Verification items for this drawing (mm, ordinates from the low corner). A direction names the side the tool comes from. Give positions to 0.01 mm unless a question says otherwise; leave off trailing zeros. Order: outer loops, then holes, each group sorted by start corner. A loop starts at its lowest first (then second) coordinate and runs counter-clockwise, first axis right, second up.
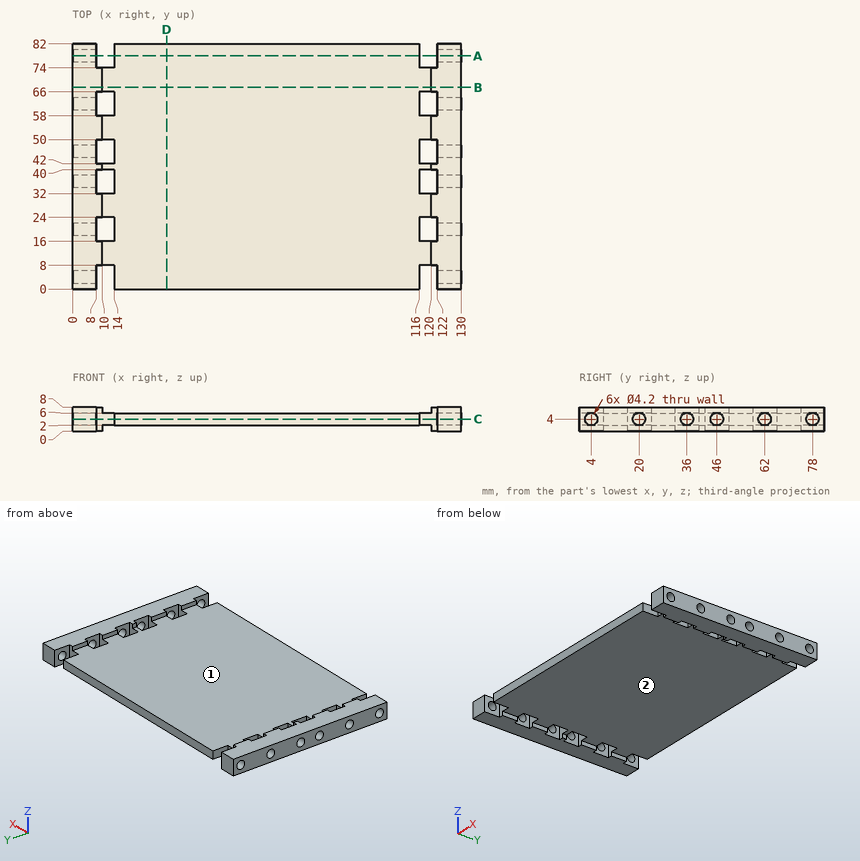
Q1. Cross-section at A-A, the plane y = 78. Record the boundary of the cut face in (x, z), and give its area (3 significant figures).
Q2. Thickness scan on L1, parallel to X at y = 49, z = 2.5; L2, parallel to Y at x = 10.5, z = 4; L3, parallel to X at y = 44, z = 6.5. Record the ranges inside material, lowest first.
Q3. Gauge pin test, flat ends, axial feed: P1, Ø4.5, axis at y = 61, z = 5, coming from the +X side; P2, Ø12, axis at x = 41, y = 22.5, coming from the +Z side; P3, Ø3, axis at y = 20, z = 3.5, coming from the -X side; P4, Ø3, axis at x = 11, z = 2.5, coming from the +Y side. Record the tip position at first contact, or that the pin passes through.
Q4. Cross-section at C-C, the plane z = 4. Give the number of separate pieces and of enclosed holes in the cut face, and give its area (3 significant figures).
Q5. Access from +Z, -Z, +X, -X, +Y, -Y to the whole of each face (thin tool, end or side, straight path). Record for the marked faces 1 and 2.
Q6. Cross-section at B-B, the plane y = 67.5. Record the boundary of the cut face in (x, z).
Q7. Cross-section at D-D, the plane x = 31.5. Record the boundary of the cut face in (y, z).
Answers follow:
1. outline: (0, 0) - (8, 0) - (8, 1.9) - (0, 1.9) - close; (0, 6.1) - (8, 6.1) - (8, 8) - (0, 8) - close; (14, 2) - (116, 2) - (116, 6) - (14, 6) - close; (122, 0) - (130, 0) - (130, 1.9) - (122, 1.9) - close; (122, 6.1) - (130, 6.1) - (130, 8) - (122, 8) - close
1. area: 469 mm2
2. L1: x = 0 to 8, 14 to 116, 122 to 130
2. L2: y = 8 to 16, 24 to 32, 40 to 42, 50 to 58, 66 to 74
2. L3: x = 0 to 8, 122 to 130
3. P1: stops at x = 130
3. P2: stops at z = 6
3. P3: stops at x = 14
3. P4: stops at y = 74
4. separate pieces: 5
4. enclosed holes: 0
4. area: 9,680 mm2
5. face 1: +Z, +Y, -Y
5. face 2: -Z, +Y, -Y
6. outline: (0, 0) - (10, 0) - (10, 2) - (120, 2) - (120, 0) - (130, 0) - (130, 8) - (120, 8) - (120, 6) - (10, 6) - (10, 8) - (0, 8) - close
7. outline: (0, 2) - (82, 2) - (82, 6) - (0, 6) - close
